Autodesk Inventor part; units mm, degrees
ref_plane "YZ Plane" through (0, 0, 0) normal (1, 0, 0) x (0, 1, 0)
ref_plane "XZ Plane" through (0, 0, 0) normal (0, 1, 0) x (-1, 0, 0)
ref_plane "XY Plane" through (0, 0, 0) normal (0, 0, 1) x (1, 0, 0)
sketch "Эскиз1" plane through (0, 0, 0) normal (0, 1, 0) x (-1, 0, 0)
  line L0 (500, -300) -> (500, 500)
  line L1 (500, 500) -> (-300, 500)
  line L2 (500, -300) -> (-300, -300)
  line L3 (-300, -300) -> (-300, 500)
  point P0 (0, 0)
  point P1 (-300, 300)
extrude "Выдавливание1" add sketch "Эскиз1" along normal blind 10
sketch "Эскиз3" plane through (0, 10, 0) normal (0, 1, 0) x (1, 0, 0)
  circle A0 centre (-203.3931, -99.1972) radius 75
  point P0 (0, 0)
  dimension "d6" = 150
extrude "Выдавливание2" cut sketch "Эскиз3" against normal blind 754.25
sketch "Эскиз4" plane through (0, 10, 0) normal (0, 1, 0) x (1, 0, 0)
  circle A0 centre (198.405, -395.8751) radius 25
  circle A1 centre (198.405, -285.8751) radius 25
  circle A2 centre (198.405, -65.8751) radius 25
  circle A3 centre (198.405, -175.8751) radius 25
  point P0 (0, 0)
  dimension "d9" = 50
  dimension "d10" = 50
  dimension "d11" = 50
  dimension "d12" = 50
  dimension "d15" = 110
  dimension "d16" = 110
  dimension "d17" = 110
extrude "Выдавливание3" cut sketch "Эскиз4" against normal blind 754.25
properties part number "ОСНОВАФАНЕРА" material "Пиломатериалы — ламинированный шпон"
The model under review builds one solid part; all positions refer to its coordinate system, in mm. Round coordinates to 2 decimals unless told otherwise and drop trailing zeros. Loops run counter-clockwise (first coordinate to the right, second up) from the corner with the lowest first, then second, coordinate; pieces in that order, holes last. Notation, with made-up numbers: M 36.5,19 L 66.5,19 A18 cw 66.5,31 Z; hole C -28.5,30.25 d9. An arc over 180 degrees is marked long. Put each result on its own line as item: value.
Q1. To check wall thickness, follow L1, parallel to X at y = 5, z = 192; L2, parallel to X at y = 9.5, z = 379.5; L3, parallel to Z at x = -166, y = 9. State the ranges of each line that lie inside material, in increasing order.
Result set:
L1: x = -500 to 179.3, 217.51 to 300
L2: x = -500 to 179.51, 217.3 to 300
L3: z = -300 to 34.18, 164.21 to 500
Q2. For pin 1 (1 mm diameter, centred on x = 213.5, z = -106, fed in from -Y), flat-tipped, find the tip position at first contact; note if it passes through.
Result set:
pin 1: stops at y = 0
Q3. Consider section A-A, the plane y = 3. Give the boundary of the cut face in (x, z) (3 decimals), then the cut area to 3 significant figures.
Result set:
outline: M -500,-300 L 300,-300 L 300,500 L -500,500 Z; hole C -203.393,99.197 d150; hole C 198.405,65.875 d50; hole C 198.405,175.875 d50; hole C 198.405,285.875 d50; hole C 198.405,395.875 d50
area: 614,000 mm²
